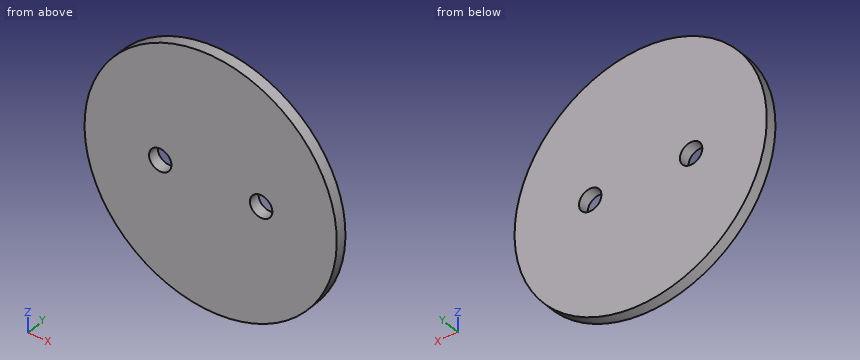
from build123d import *

# Parameters (mm, degrees)
SKETCH1_R           = 4.5
BOSS_EXTRUDE1_DEPTH = 0.5
SKETCH2_R           = 0.5
CUT_EXTRUDE1_DEPTH  = 7.383572667
BOSS_EXTRUDE2_START = -0.5
SKETCH3_R           = 5.625
SKETCH3_R_2         = 4.5
BOSS_EXTRUDE2_DEPTH = 0.5


with BuildPart() as part:
    # Sketch1 → Boss-Extrude1 (new body)
    with BuildSketch(Plane(origin=(0, 0, 0), x_dir=(1, 0, 0), z_dir=(0, 1, 0))):
        with Locations(Location((0, 0, 0), (0, 0, 270))):
            Circle(SKETCH1_R)
    extrude(amount=BOSS_EXTRUDE1_DEPTH)

    # Sketch2 → Cut-Extrude1 (cut, through all)
    with BuildSketch(Plane(origin=(0, 0.5, 0), x_dir=(1, 0, 0), z_dir=(0, 1, 0))):
        with Locations(Location((-2.25, 0, 0), (0, 0, 270))):
            Circle(SKETCH2_R)
        with Locations(Location((2.25, 0, 0), (0, 0, 270))):
            Circle(SKETCH2_R)
    extrude(amount=-CUT_EXTRUDE1_DEPTH, mode=Mode.SUBTRACT)

    # Sketch3 → Boss-Extrude2 (add)
    with BuildSketch(Plane(origin=(0, 0.5, 0), x_dir=(1, 0, 0), z_dir=(0, 1, 0)).offset(BOSS_EXTRUDE2_START)):
        with Locations(Location((0, 0, 0), (0, 0, 270))):
            Circle(SKETCH3_R)
        Circle(SKETCH3_R_2, mode=Mode.SUBTRACT)
    extrude(amount=BOSS_EXTRUDE2_DEPTH)


solid = part.part
Work out the finished part from the listing and answer in its coordinate system (mm). Coordinates: 2 decimals unless noted, no trailing zeros. Write each loop counter-clockwise with the first axis right and the second up, starting at its lowest first coordinate (ties: lowest second). Pieces come first, ordered by that corner, then holes. Notation, with made-up numbers: M 45.25,20 L 95.25,20 A20 cw 95.25,57 Z; hole C 17,-23 d4. An arc over 180 degrees is marked long. Write item = value, one per line.
1. Straight lines are drawn through the part: line 1 (X direction, y = 0.25, z = 0) (3 decimals); line 2 (Z direction, x = 2, y = 0.4); line 3 (Z direction, x = -4, y = 0.1). For each, find the intervals that lie inside material, in ascending order. Write a range as from..to.
Solution:
line_1 = -5.625..-2.75, -1.75..1.75, 2.75..5.625
line_2 = -5.26..-0.43, 0.43..5.26
line_3 = -3.95..3.95
2. The part is cut by section C-C (y = 0.4). Determine the outline of the cut face in (x, z) (3 decimals), then the cut area to 3 significant figures.
Solution:
outline = C 0,0 d11.25; hole C -2.25,0 d1; hole C 2.25,0 d1
area = 97.8 mm2
3. The part is cut by section B-B (x = -2.25). Determine the outline of the cut face in (y, z).
Solution:
outline = M 0,-5.16 L 0.5,-5.16 L 0.5,-0.5 L 0,-0.5 Z; M 0,0.5 L 0.5,0.5 L 0.5,5.16 L 0,5.16 Z
4. The part is cut by section D-D (x = 2.5). Determine the outline of the cut face in (y, z), then the cut area to 3 significant figures.
Solution:
outline = M 0,-5.04 L 0.5,-5.04 L 0.5,-0.43 L 0,-0.43 Z; M 0,0.43 L 0.5,0.43 L 0.5,5.04 L 0,5.04 Z
area = 4.61 mm2
5. The part is cut by section A-A (z = 0). Determine the outline of the cut face in (x, y) (3 decimals), then the cut area to 4 significant figures.
Solution:
outline = M -5.625,0 L -2.75,0 L -2.75,0.5 L -5.625,0.5 Z; M -1.75,0 L 1.75,0 L 1.75,0.5 L -1.75,0.5 Z; M 2.75,0 L 5.625,0 L 5.625,0.5 L 2.75,0.5 Z
area = 4.625 mm2
